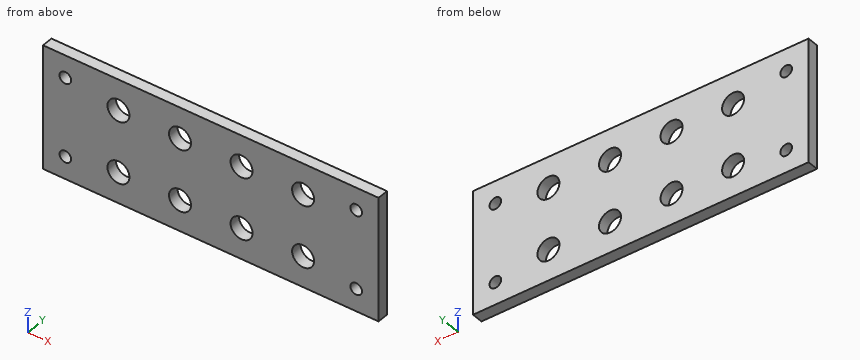
Autodesk Inventor part; units mm, degrees
ref_plane "YZ Plane" through (0, 0, 0) normal (1, 0, 0) x (0, 1, 0)
ref_plane "XZ Plane" through (0, 0, 0) normal (0, 1, 0) x (-1, 0, 0)
ref_plane "XY Plane" through (0, 0, 0) normal (0, 0, 1) x (1, 0, 0)
sketch "Sketch1" plane through (0, 0, 0) normal (0, 1, 0) x (-1, 0, 0)
  circle A0 centre (0, 0) radius 6.25
  line L0 (0, 0) -> (0, 25.4) construction
  line L1 (0, 0) -> (-101.6, 0) construction
  circle A1 centre (0, 35) radius 6.25
  circle A2 centre (-35, 0) radius 6.25
  circle A3 centre (-35, 35) radius 6.25
  circle A4 centre (-70, 0) radius 6.25
  circle A5 centre (-70, 35) radius 6.25
  circle A6 centre (-105, 0) radius 6.25
  circle A7 centre (-105, 35) radius 6.25
  line L2 (42.9, -17.5) -> (-147.9, -17.5)
  line L3 (-147.9, -17.5) -> (-147.9, 52.5)
  line L4 (-147.9, 52.5) -> (42.9, 52.5)
  line L5 (42.9, 52.5) -> (42.9, -17.5)
  circle A8 centre (30.2, -4.8) radius 3.302
  circle A9 centre (-135.2, -4.8) radius 3.302
  circle A10 centre (-135.2, 39.8) radius 3.302
  circle A11 centre (30.2, 39.8) radius 3.302
  dimension "d0" = 12.5
  dimension "d1" = 25.4
  dimension "d2" = 101.6
  dimension "d5" = 35
  dimension "d8" = 35
  dimension "d11" = 42.9
  dimension "d12" = 42.9
  dimension "d13" = 17.5
  dimension "d14" = 17.5
  dimension "d15" = 6.604
  dimension "d16" = 12.7
  dimension "d17" = 12.7
  dimension "d18" = 6.604
  dimension "d19" = 12.7
  dimension "d20" = 6.604
  dimension "d21" = 12.7
  dimension "d22" = 6.604
extrude "Extrusion1" add sketch "Sketch1" along normal blind 6.35
equation "\"d14\" = 0.5 * d5"
properties part number "SequenceMachine_VialPlate"
Here's how the part is built. I have some questions about the finished solid (model axes, mm). Round coordinates to 2 decimals unless told otherwise and drop trailing zeros. Order: outer loops, then holes, each group sorted by start corner. A loop starts at its lowest first (then second) coordinate and runs counter-clockwise, first axis right, second up. Notation, with made-up numbers: (14, 35) -> (70, 35) arc R15 cw to (70, 58) -> close; hole circle Ø4 at (7, -0.5). An arc over 180 degrees is marked (long way). Use a Markdown table: item, result. Add a question column.
(1) I need wall thicknesses on line 1 along Z through (x, y) = (-30.2, 2.75); line 2 along Z through (x, y) = (35, 1.5); line 3 along X through (y, z) = (6.25, 42.5). Which ranges of each line are inside material? Lowest first, please.
(2) Suppose I cut it at C-C, the plane x = 135.2. Please give me the cut outline in (y, z).
(3) Suppose I cut it at B-B, the plane y = 4.5. Count the separate pieces of the cut face and the enclosed holes in it, and give its area (3 significant figures).
(4) Suppose I cut it at A-A, the plane x = 0. Please give me the cut outline in (y, z).
(5) For pin 1 Ø7.5 at (x, z) = (105, 0) entering from +Y, with a flat end and sliding along its axis, tell me the tip position at first contact or that it passes through.
Verdict:
| question | item | result |
|---|---|---|
| 1 | line 1 | -17.5 to -8.1, -1.5 to 36.5, 43.1 to 52.5 |
| 1 | line 2 | -17.5 to -6.25, 6.25 to 28.75, 41.25 to 52.5 |
| 1 | line 3 | -42.9 to -32.1, -28.3 to 133.3, 137.1 to 147.9 |
| 2 | outline | (0, -17.5) -> (6.35, -17.5) -> (6.35, -8.1) -> (0, -8.1) -> close; (0, -1.5) -> (6.35, -1.5) -> (6.35, 36.5) -> (0, 36.5) -> close; (0, 43.1) -> (6.35, 43.1) -> (6.35, 52.5) -> (0, 52.5) -> close |
| 3 | separate pieces | 1 |
| 3 | enclosed holes | 12 |
| 3 | area | 12,200 mm2 |
| 4 | outline | (0, -17.5) -> (6.35, -17.5) -> (6.35, -6.25) -> (0, -6.25) -> close; (0, 6.25) -> (6.35, 6.25) -> (6.35, 28.75) -> (0, 28.75) -> close; (0, 41.25) -> (6.35, 41.25) -> (6.35, 52.5) -> (0, 52.5) -> close |
| 5 | pin 1 | through |
